The model under review builds one solid part; all positions refer to its coordinate system, in mm. Face numbers are marked on the shaded views. A direction names the side the tool comes from. Coordinates: 2 decimals unless noted, no trailing zeros. Write each loop counter-clockwise with the first axis right and the second up, starting at its lowest first coordinate (ties: lowest second). Pieces come first, ordered by that corner, then holes.
1) Add section B-B, the plane x = 4. State the section outline as (y, z) points.
2) Machinability: for the marked faces 1 and 2, which of the approach directions +Z, -Z, +X, -X, +Y, -Y give a long, thin tool a straight path to every point of the face, cutting with its end or side? Answer none if there is none.
3) Add section D-D, the plane x = -5.25. State the section outline as (y, z) points, then the cut area to 3 significant figures.
4) Add section C-C, the plane z = -11.5. Give the number of separate pieces and of enclosed holes in the cut face, then the cut area to 3 significant figures.
5) For P1, Ø3, axis at y = -30.5, z = -8, coming from the +X side; P2, Ø1.5, axis at y = 41.5, z = -2.5, coming from the -X side; P3, Ø4, axis at x = -3.5, z = -8, coming from the +Y side, all flat-tipped, find the tip position at first contact; note any pin that passes through.
6) Add section A-A, the plane y = -45. State the section outline as (x, z) points, then the cut area to 3 significant figures.
7) Mouldability with a two-part tool opening along X and no side actions: class the marked faces 3, 4, 5 and 6 as released by +X, released by -X, zero draft, split by the parting line, or undercut.
8) For line 1 (Z direction, x = -2.75, y = 54.5); line 2 (X direction, y = -40.5, z = -9); line 3 (Z direction, x = 3.25, y = 25), list the stretches that pass through material, from the lowest coordinate up.
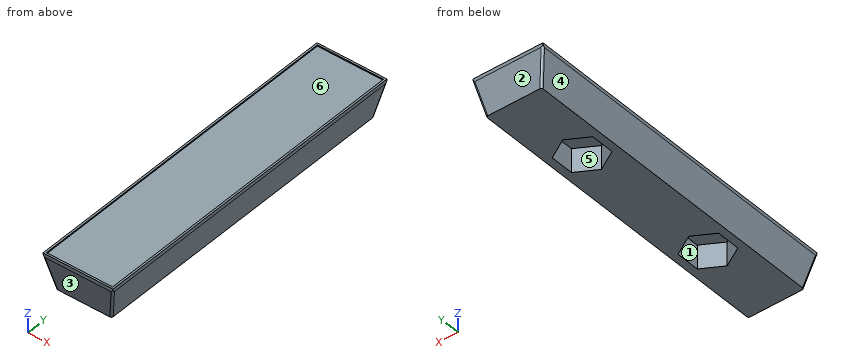
from build123d import *

# Parameters (mm, degrees)
F1_W     = 29.5
F1_H     = 140.5
F1_W_2   = 27.9
F1_H_2   = 138.9
F2_DEPTH = 0.5
F3_DEPTH = 15
F4_SIZE2 = 14
F4_SIZE  = 3
F5_R     = 0.8
F7_DEPTH = 10


with BuildPart() as f2:
    # F1 (on Top) → F2 (new body)
    with BuildSketch(Plane.XY):
        Rectangle(F1_W, F1_H)
        Rectangle(F1_W_2, F1_H_2, mode=Mode.SUBTRACT)
    extrude(amount=F2_DEPTH)

    # F1 (on Top) → F3 (join)
    with BuildSketch(Plane.XY):
        Rectangle(F1_W, F1_H)
        Rectangle(F1_W_2, F1_H_2, mode=Mode.SUBTRACT)
        Rectangle(F1_W_2, F1_H_2)
    extrude(amount=-F3_DEPTH)

    # F4
    f4_edges = [f2.edges().sort_by_distance(p)[0] for p in [
        (0, -70.25, -15),
        (14.75, 0, -15),
        (0, 70.25, -15),
        (-14.75, 0, -15),
    ]]
    f4_side = f2.faces().sort_by_distance((0, 0, -15))[0]
    chamfer(f4_edges, length=F4_SIZE, length2=F4_SIZE2, reference=f4_side)

    # F5
    f5_edges = [f2.edges().sort_by_distance(p)[0] for p in [
        (13.25, 68.75, -8),
        (-13.25, 68.75, -8),
        (13.25, -68.75, -8),
        (-13.25, -68.75, -8),
    ]]
    fillet(f5_edges, radius=F5_R)

    # F6 (on face) → F7 (cut)
    with BuildSketch(Plane(origin=(0, 0, -15), x_dir=(1, 0, 0), z_dir=(0, 0, -1))):
        Polygon((-8.55, 37.1863448016), (-8.55, 27.3136551984), (0, 22.3773103969), (8.55, 27.3136551984), (8.55, 37.1863448016), (0, 42.1226896031), align=None)
        Polygon((-8.55, -37.1863448016), (0, -42.1226896031), (8.55, -37.1863448016), (8.55, -27.3136551984), (0, -22.3773103969), (-8.55, -27.3136551984), align=None)
    extrude(amount=-F7_DEPTH, mode=Mode.SUBTRACT)


solid = f2.part
Geometry results:
1. outline: (-70.25, -1) - (-67.25, -15) - (-39.81, -15) - (-39.81, -5) - (-24.69, -5) - (-24.69, -15) - (24.69, -15) - (24.69, -5) - (39.81, -5) - (39.81, -15) - (67.25, -15) - (70.25, -1) - (70.25, 0.5) - (69.45, 0.5) - (69.45, 0) - (-69.45, 0) - (-69.45, 0.5) - (-70.25, 0.5) - close
2. face 1: -Z
2. face 2: -Z, +X, -X, +Y
3. outline: (-70.25, -1) - (-67.25, -15) - (-39.09, -15) - (-39.09, -5) - (-25.41, -5) - (-25.41, -15) - (25.41, -15) - (25.41, -5) - (39.09, -5) - (39.09, -15) - (67.25, -15) - (70.25, -1) - (70.25, 0.5) - (69.45, 0.5) - (69.45, 0) - (-69.45, 0) - (-69.45, 0.5) - (-70.25, 0.5) - close
3. area: 1,790 mm2
4. separate pieces: 1
4. enclosed holes: 2
4. area: 2,890 mm2
5. P1: stops at x = 13.57
5. P2: stops at x = -14.59
5. P3: stops at y = 69.18
6. outline: (-14.75, -1) - (-11.75, -15) - (11.75, -15) - (14.75, -1) - (14.75, 0.5) - (13.95, 0.5) - (13.95, 0) - (-13.95, 0) - (-13.95, 0.5) - (-14.75, 0.5) - close
6. area: 401 mm2
7. face 3: zero draft
7. face 4: released by -X
7. face 5: undercut
7. face 6: undercut
8. line 1: z = -15 to 0
8. line 2: x = -13.04 to -2.81, 2.81 to 13.04
8. line 3: z = -5 to 0
